For this review, take the finished solid that the model builds, in its own axes (mm). A direction names the side the tool comes from. Coordinates: 2 decimals unless noted, no trailing zeros. Loops run counter-clockwise (first coordinate to the right, second up) from the corner with the lowest first, then second, coordinate; pieces in that order, holes last. Notation, with made-up numbers: (26, 9) -> (70, 9) arc R28 cw to (70, 48) -> close; hole circle Ø9 at (28, -30). An arc over 180 degrees is marked (long way). Use a Markdown table: item, result.
from build123d import *

# Parameters (mm, degrees)
PAH1_SIZE = 0.5


with BuildPart() as part:
    # Çizim1 → Döndür1 (revolve)
    with BuildSketch(Plane.XY, mode=Mode.PRIVATE) as d_nd_r1_sk:
        Polygon((1.89, 4), (35, 4), (51, 8), (129, 8), (144, 5), (154.5, 5), (156.49, 5), (156.49, 3.5), (198.5, 3.5), (199.49, 3.5), (199.49, 0), (198.5, 0), (1.89, 0), align=None)
    revolve(d_nd_r1_sk.sketch.rotate(Axis((1.89, 0, 0), (1, 0, 0)), 90), axis=Axis((1.89, 0, 0), (1, 0, 0)))

    # Pah1
    pah1_edges = [part.edges().sort_by_distance(p)[0] for p in [
        (1.89, 0, -4),
    ]]
    chamfer(pah1_edges, length=PAH1_SIZE)


solid = part.part
(1) For line 1 along Y through (x, z) = (146, 0); line 2 along Z through (x, y) = (96, 0.5); line 3 along Y through (x, z) = (91.5, -4.5), list the stretches that pass through material, from the lowest coordinate up.
Found:
| item | result |
|---|---|
| line 1 | y = -5 to 5 |
| line 2 | z = -7.98 to 7.98 |
| line 3 | y = -6.61 to 6.61 |
(2) Take a section at D-D on x = 20. Write out the cut boundary in (y, z), plus the area to 3 significant figures.
Found:
| item | result |
|---|---|
| outline | circle Ø8 at (0, 0) |
| area | 50.3 mm^2 |
(3) For faces 1 (the face through (18.923, 3.905, -0.867)), 2 (the face through (199.49, 0, 0)), 3 (the face through (156.49, 3.3, 2.2)), list the 3-axis set-ups (+Z, -Z, +X, -X, +Y, -Y) from which the entire face can be reached by the end or side of a thin tool; tool diameter is ignored.
Found:
| item | result |
|---|---|
| face 1 | -X |
| face 2 | +Z, -Z, +X, +Y, -Y |
| face 3 | +X |
(4) Take a section at A-A on z = 0. Write out the cut boundary in (x, y), plus the area to 3 significant figures.
Found:
| item | result |
|---|---|
| outline | (1.89, -3.5) -> (2.39, -4) -> (35, -4) -> (51, -8) -> (129, -8) -> (144, -5) -> (156.49, -5) -> (156.49, -3.5) -> (199.49, -3.5) -> (199.49, 3.5) -> (156.49, 3.5) -> (156.49, 5) -> (144, 5) -> (129, 8) -> (51, 8) -> (35, 4) -> (2.39, 4) -> (1.89, 3.5) -> close |
| area | 2,330 mm^2 |
(5) For pin 1 Ø1 at (x, z) = (156.5, -3.5) entering from +Y; pin 2 Ø5 at (x, z) = (82.5, -4) entering from -Y; pin 3 Ø6 at (y, z) = (-5, 1.5) entering from -X; pin 4 Ø6 at (x, y) = (150.5, 3) entering from +Z, all flat-tipped, find the tip position at first contact; note any pin that passes through.
Found:
| item | result |
|---|---|
| pin 1 | stops at y = 4 |
| pin 2 | stops at y = -7.86 |
| pin 3 | stops at x = 1.89 |
| pin 4 | stops at z = 5 |
(6) Take a section at C-C on x = 75. Write out the cut boundary in (y, z).
Found:
| item | result |
|---|---|
| outline | circle Ø16 at (0, 0) |
